from build123d import *

# Parameters (mm, degrees)
SKETCH015_W         = 60
SKETCH015_H         = 50
PAD005_DEPTH        = 15
HOLE006_D           = 2.8
HOLE006_DEPTH       = 25
HOLE006_CBORE_D     = 6
HOLE006_CBORE_DEPTH = 10
SKETCH018_R         = 2.15
HOLE007_DEPTH       = 25
FILLET008_R         = 0.5
FILLET009_R         = 2


with BuildPart() as part:
    # Sketch015 → Pad005 (new body)
    with BuildSketch(Plane.XY):
        Rectangle(SKETCH015_W, SKETCH015_H)
    extrude(amount=PAD005_DEPTH)

    # Hole006
    with Locations(Plane.XY.offset(15)):
        with Locations((23, 18), (23, -18)):
            hole006 = CounterBoreHole(HOLE006_D / 2, HOLE006_CBORE_D / 2, HOLE006_CBORE_DEPTH, depth=HOLE006_DEPTH)

    # Mirrored009: Hole006 across Sketch016 V_Axis
    add(hole006.mirror(Plane(origin=(0, 0, 15), x_dir=(0, 0, 1), z_dir=(1, 0, 0))), mode=Mode.SUBTRACT)

    # Sketch018 → Hole007 (cut)
    with BuildSketch(Plane.XY.offset(15)):
        with Locations((14, 11)):
            Circle(SKETCH018_R)
    hole007 = extrude(amount=-HOLE007_DEPTH, mode=Mode.SUBTRACT)

    # Mirrored011: Hole007 across Sketch018 V_Axis
    add(hole007.mirror(Plane(origin=(0, 0, 15), x_dir=(0, 0, 1), z_dir=(1, 0, 0))), mode=Mode.SUBTRACT)

    # Fillet008
    fillet008_edges = [part.edges().sort_by_distance(p)[0] for p in [
        (-30, -25, 7.5),
        (30, -25, 7.5),
        (30, 25, 7.5),
        (-30, 25, 7.5),
    ]]
    fillet(fillet008_edges, radius=FILLET008_R)

    # Fillet009
    fillet009_edges = [part.edges().sort_by_distance(p)[0] for p in [
        (0, 25, 15),
        (-30, 0, 15),
        (30, 0, 15),
        (0, -25, 15),
    ]]
    fillet(fillet009_edges, radius=FILLET009_R)


solid = part.part
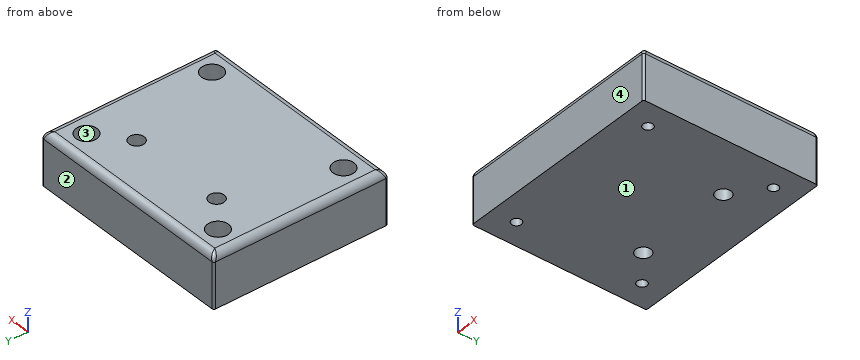
Input: part model. Units: mm. Frame: model coordinates. Face numbers are marked on the shaded views. Coordinates: 2 decimals unless noted, no trailing zeros. Order: outer loops, then holes, each group sorted by start corner. A loop starts at its lowest first (then second) coordinate and runs counter-clockwise, first axis right, second up.
1. Cut plane D-D, the plane x = -15. Return loops of the section in (y, z), plus the area to 3 significant figures.
Checked values:
outline: (-25, 0) - (9.1, 0) - (9.1, 15) - (-23, 15) arc R2 ccw to (-25, 13) - close; (12.9, 0) - (25, 0) - (25, 13) arc R2 ccw to (23, 15) - (12.9, 15) - close
area: 691 mm2
2. Ray query, line 1 along Y through (x, z) = (23, 1.85); line 2 along Y through (x, z) = (21, 10.5); line 3 along Y through (x, z) = (-14, 6.5). Return the intervals inside material, ascending.
Checked values:
line 1: y = -25 to -19.4, -16.6 to 16.6, 19.4 to 25
line 2: y = -25 to -20.24, -15.76 to 15.76, 20.24 to 25
line 3: y = -25 to 8.85, 13.15 to 25
3. Cut plane A-A, the plane z = 10. Return loops of the section in (x, y).
Checked values:
outline: (-30, -24.5) arc R0.5 ccw to (-29.5, -25) - (29.5, -25) arc R0.5 ccw to (30, -24.5) - (30, 24.5) arc R0.5 ccw to (29.5, 25) - (-29.5, 25) arc R0.5 ccw to (-30, 24.5) - close; hole circle Ø6 at (-23, -18); hole circle Ø6 at (-23, 18); hole circle Ø4.3 at (-14, 11); hole circle Ø4.3 at (14, 11); hole circle Ø6 at (23, -18); hole circle Ø6 at (23, 18)
4. Cut plane B-B, the plane y = 18. Return loops of the section in (x, z), plus the area to 3 significant figures.
Checked values:
outline: (-30, 0) - (-24.4, 0) - (-24.4, 5) - (-26, 5) - (-26, 15) - (-28, 15) arc R2 ccw to (-30, 13) - close; (-21.6, 0) - (21.6, 0) - (21.6, 5) - (20, 5) - (20, 15) - (-20, 15) - (-20, 5) - (-21.6, 5) - close; (24.4, 0) - (30, 0) - (30, 13) arc R2 ccw to (28, 15) - (26, 15) - (26, 5) - (24.4, 5) - close
area: 750 mm2
5. Cut plane C-C, the plane x = -23. Return loops of the section in (y, z), plus the area to 3 significant figures.
Checked values:
outline: (-25, 0) - (-19.4, 0) - (-19.4, 5) - (-21, 5) - (-21, 15) - (-23, 15) arc R2 ccw to (-25, 13) - close; (-16.6, 0) - (16.6, 0) - (16.6, 5) - (15, 5) - (15, 15) - (-15, 15) - (-15, 5) - (-16.6, 5) - close; (19.4, 0) - (25, 0) - (25, 13) arc R2 ccw to (23, 15) - (21, 15) - (21, 5) - (19.4, 5) - close
area: 600 mm2
6. Draft query along Y for the marked faces 1, 2, 3 and 4. Return one class per face: +Y half, -Y half, draft (parallel to the pull), parting line (faces both ways), or undercut.
Checked values:
face 1: draft
face 2: +Y half
face 3: undercut
face 4: -Y half
7. Contact query for flat-ended pins moving along their axis: P1, Ø3, axis at x = -23, y = -18, coming from the +Z side; P2, Ø3.5, axis at x = 23, y = -18, coming from the -Z side. Output: stop coordinate, or through.
Checked values:
P1: stops at z = 5
P2: stops at z = 0
